Input: part model. Units: mm. Frame: model coordinates. A direction names the side the tool comes from. Coordinates: 2 decimals unless noted, no trailing zeros. Loops run counter-clockwise (first coordinate to the right, second up) from the corner with the lowest first, then second, coordinate; pieces in that order, holes last.
Item 1: Reachability of faces 5 (the cylindrical face through (-10.425, -0.175, -25.422)), 6 (the cylindrical face through (84.183, 11.865, -19.58)), 7 (the flat face through (-10, 12.5, -32)) from +Z, -Z, +X, -X, +Y, -Y: full face, straight path, thin tool, end or side. Return the list, or none.
Item 2: Section A-A on x = -13.5. Return loops of the section in (y, z).
Item 3: Pull-direction query (Y, two-part tool) for faces 1 (the cylindrical face through (56.823, -7.91, -60.14)), 2 (the cylindrical face through (92.44, -19.05, -33.02)), 3 (the flat face through (57, -10, -70)), 4 (the flat face through (-10, -12.5, -32)); classes: released by +Y, released by -Y, zero draft, split by the parting line, or undercut.
Item 4: Contact query for flat-ended pins moving along their axis: P1, Ø8, axis at x = -12, y = 3.5, coming from the +Z side; P2, Ø1.5, axis at x = 11.5, z = -16.5, coming from the -Y side; P3, Ø10, axis at x = 24, z = -56, coming from the -Y side. Output: stop coordinate, or through.
Item 5: Section C-C on z = -24. Return loops of the section in (x, y).
Item 6: Ray query, line 1 along Y through (x, z) = (45.5, -35); line 2 along Y through (x, z) = (-8, -19); line 3 along X through (y, z) = (29.5, -9.5). Return the intervals inside material, ascending.
```python
from build123d import *

# Parameters (mm, degrees)
F1_DEPTH       = 12.5
F2_R           = 49.7287092038
F3_DEPTH       = 70
F5_DEPTH       = 10
F8_D           = 26
F8_CBORE_D     = 79
F8_CBORE_DEPTH = 60
F9_R           = 5
F10_R          = 4.99999


# Not quite as in the source:
# - a fillet or chamfer is up to 0.001 mm smaller than in the source, because OpenCascade refuses the exact size
# - a feature names something its author has since deleted; it is built from what else it names


with BuildPart() as f1:
    # F0 (on Front) → F1 (new body, symmetric)
    with BuildSketch(Plane.XZ):
        with BuildLine():
            Line((0, -70), (0, 0))
            Line((0, 0), (-23, 0))
            Line((-23, 0), (-23, -13))
            ThreePointArc((-23, -13), (-10.4224046937, -25.699410108), (-23, -38.398820216))
            Line((-23, -38.398820216), (-23, -51.398820216))
            Line((-23, -51.398820216), (0, -70))
        make_face()
    extrude(amount=F1_DEPTH, both=True)

    # F2 (on Top) → F3 (join)
    with BuildSketch(Plane.XY):
        with Locations((46.5068519115, 0)):
            Circle(F2_R)
    extrude(amount=-F3_DEPTH)

    # F2 (on Top) → F5 (join)
    with BuildSketch(Plane.XY):
        with Locations((46.5068519115, 0)):
            Circle(F2_R)
    extrude(amount=F5_DEPTH)

    # F8 (through all)
    with Locations(Plane.XY.offset(10)):
        with Locations((46.5068519115, 0)):
            CounterBoreHole(F8_D / 2, F8_CBORE_D / 2, F8_CBORE_DEPTH)

    # F9
    f9_edges = [f1.edges().sort_by_distance(p)[0] for p in [
        (-3.221857, 0, 10),
    ]]
    fillet(f9_edges, radius=F9_R)

    # F10 (radius 5 in the source; OpenCascade refuses exactly that, so slightly less here)
    f10_edges = [f1.edges().sort_by_distance(p)[0] for p in [
        (-1.625201, 12.5, -34.342812),
        (-1.625201, -12.5, -34.342812),
        (-3.221857, 0, 0),
    ]]
    fillet(f10_edges, radius=F10_R)


solid = f1.part
```
Results found:
1. face 5: -X, +Y, -Y
1. face 6: +Z
1. face 7: +Z, -Z, -X, +Y
2. outline: (-12.5, -59.08) - (12.5, -59.08) - (12.5, -33.99) - (-12.5, -33.99) - close; (-12.5, -17.41) - (12.5, -17.41) - (12.5, 0) - (-12.5, 0) - close
3. face 1: undercut
3. face 2: split by the parting line
3. face 3: zero draft
3. face 4: released by -Y
4. P1: stops at z = 0
4. P2: stops at y = -36.05
4. P3: stops at y = -46.55
5. outline: (-10.54, -12.5) - (-5.35, -12.5) arc R5 cw to (-0.61, -15.9) arc R49.73 ccw (long way) to (-0.61, 15.9) arc R5 cw to (-5.35, 12.5) - (-10.54, 12.5) - close; hole circle Ø79 at (46.51, 0)
6. line 1: y = -49.72 to -39.49, 39.49 to 49.72
6. line 2: y = -12.5 to 12.5
6. line 3: x = 6.47 to 20.24, 72.77 to 86.54
